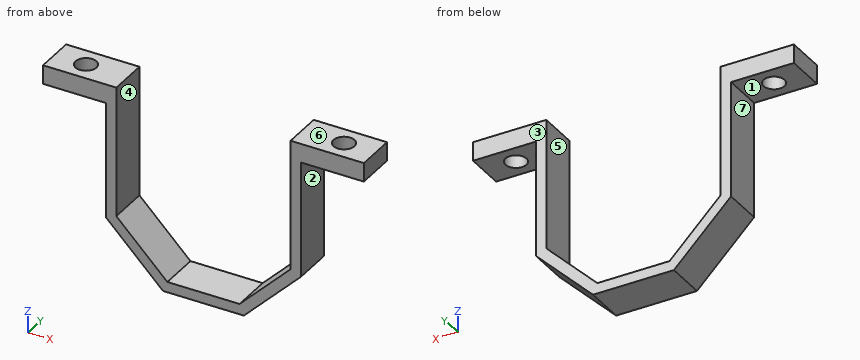
from build123d import *

# Parameters (mm, degrees)
BOSS_EXTRUDE1_DEPTH = 9.5
SKETCH3_R           = 2.5
CUT_EXTRUDE1_DEPTH  = 9.5


with BuildPart() as part:
    # Sketch2 → Boss-Extrude1 (new body)
    with BuildSketch(Plane(origin=(0, 0, 0), x_dir=(1, 0, 0), z_dir=(0, 1, 0))):
        Polygon((-9.650154056, 23.297532801), (-23.297532801, 9.650154056), (-23.297532801, -9.650154056), (-23.297532801, -18.047532806), (-38.297532801, -18.047532806), (-38.297532801, -22.547532806), (-23.297532801, -22.547532806), (-20.797532801, -22.547532806), (-20.797532801, -12.150154056), (-20.797532801, -8.61462015), (-20.797532801, 8.61462015), (-8.61462015, 20.797532801), (8.61462015, 20.797532801), (20.797532801, 8.61462015), (20.797532801, -8.61462015), (20.797532801, -12.150154056), (20.797532801, -22.547532806), (23.297532801, -22.547532806), (38.297532801, -22.547532806), (38.297532801, -18.047532806), (23.297532801, -18.047532806), (23.297532801, -9.650154056), (23.297532801, 9.650154056), (9.650154056, 23.297532801), align=None)
    extrude(amount=BOSS_EXTRUDE1_DEPTH)

    # Sketch3 → Cut-Extrude1 (cut)
    with BuildSketch(Plane(origin=(0, 0, 18.047532806), x_dir=(-1, 0, 0), z_dir=(0, 0, -1))):
        with Locations((30.797532801, 4.75)):
            Circle(SKETCH3_R)
        with Locations((-30.797532801, 4.75)):
            Circle(SKETCH3_R)
    extrude(amount=-CUT_EXTRUDE1_DEPTH, mode=Mode.SUBTRACT)


solid = part.part
Read the model definition and answer for the solid it produces. Units are mm, in the model's axes. Face numbers are marked on the shaded views. A direction names the side the tool comes from. Give positions to 0.01 mm unless a question says otherwise; leave off trailing zeros. Loops run counter-clockwise (first coordinate to the right, second up) from the corner with the lowest first, then second, coordinate; pieces in that order, holes last. Notation, with made-up numbers: (-15, -30.75) -> (13, -30.75) arc R23 cw to (13, -9.75) -> close; hole circle Ø6 at (48.25, 30). An arc over 180 degrees is marked (long way). Use a Markdown table: item, result.
Q1. Find the intervals of material crossed by line 1 along X through (y, z) = (4.5, 6); line 2 along X through (y, z) = (1.5, 18.5); line 3 along Z through (x, y) = (-3.5, 0.5), in increasing order.
Solved:
| item | result |
|---|---|
| line 1 | x = -23.3 to -20.8, 20.8 to 23.3 |
| line 2 | x = -38.3 to -20.8, 20.8 to 38.3 |
| line 3 | z = -23.3 to -20.8 |
Q2. Section B-B, the plane z = 11 is taken. Determine the outline of the cut face in (x, y), then the cut area to 3 significant figures.
Solved:
| item | result |
|---|---|
| outline | (-23.3, 0) -> (-20.8, 0) -> (-20.8, 9.5) -> (-23.3, 9.5) -> close; (20.8, 0) -> (23.3, 0) -> (23.3, 9.5) -> (20.8, 9.5) -> close |
| area | 47.5 mm^2 |
Q3. Section D-D, the plane x = -25.5 is taken. Determine the outline of the cut face in (y, z), then the cut area to 4 significant figures.
Solved:
| item | result |
|---|---|
| outline | (0, 18.05) -> (9.5, 18.05) -> (9.5, 22.55) -> (0, 22.55) -> close |
| area | 42.75 mm^2 |
Q4. Section A-A, the plane y = 4.75 is taken. Determine the outline of the cut face in (x, z).
Solved:
| item | result |
|---|---|
| outline | (-38.3, 18.05) -> (-33.3, 18.05) -> (-33.3, 22.55) -> (-38.3, 22.55) -> close; (-28.3, 18.05) -> (-23.3, 18.05) -> (-23.3, -9.65) -> (-9.65, -23.3) -> (9.65, -23.3) -> (23.3, -9.65) -> (23.3, 18.05) -> (28.3, 18.05) -> (28.3, 22.55) -> (20.8, 22.55) -> (20.8, -8.61) -> (8.61, -20.8) -> (-8.61, -20.8) -> (-20.8, -8.61) -> (-20.8, 22.55) -> (-28.3, 22.55) -> close; (33.3, 18.05) -> (38.3, 18.05) -> (38.3, 22.55) -> (33.3, 22.55) -> close |
Q5. Section C-C, the plane z = -10.5 is taken. Determine the outline of the cut face in (x, y), then the cut area to 3 significant figures.
Solved:
| item | result |
|---|---|
| outline | (-22.45, 0) -> (-18.91, 0) -> (-18.91, 9.5) -> (-22.45, 9.5) -> close; (18.91, 0) -> (22.45, 0) -> (22.45, 9.5) -> (18.91, 9.5) -> close |
| area | 67.2 mm^2 |
Q6. Determine the mould class of the marked faces 5, 6 and 7 for opening direction X: pulls with the +X half, pulls with the -X half, needs draft (parallel to the pull), parting line crosses it, or undercut.
Solved:
| item | result |
|---|---|
| face 5 | undercut |
| face 6 | needs draft |
| face 7 | pulls with the -X half |
Q7. Each of these flat-tipped pins is pushed along its axis until it touches: pin 1 (1 mm diameter, centred on x = 15.5, y = 7, fed in from -Z); pin 2 (1.5 mm diameter, centred on y = 5, z = -0.5, fed in from -X); pin 3 (5 mm diameter, centred on x = -0.5, y = 6, fed in from +Z). Where does it stop, or does it pass through?
Solved:
| item | result |
|---|---|
| pin 1 | stops at z = -17.95 |
| pin 2 | stops at x = -23.3 |
| pin 3 | stops at z = -20.8 |
Q8. A tool of negligible diameter and unlimited length cuts with its end or side. For the marked faces 1, 2, 3 and 4, from which of +Z, -Z, +X, -X, +Y, -Y can it reach the whole face along a straight path? Write none if from no direction.
Solved:
| item | result |
|---|---|
| face 1 | -Z, -X, +Y, -Y |
| face 2 | -Z, +X, +Y, -Y |
| face 3 | +Z, -Z, +X, -X, +Y |
| face 4 | +Z, +Y, -Y |
